Could you check a few things on this model? Use its own coordinates, in mm. A direction names the side the tool comes from. Give positions to 0.01 mm unless a question says otherwise; leave off trailing zeros. Write each loop counter-clockwise with the first axis right and the second up, starting at its lowest first coordinate (ties: lowest second). Pieces come first, ordered by that corner, then holes. Notation, with made-up numbers: M 10,28 L 27,28 A17 cw 27,41 Z; hole C -28.5,-35.75 d2. An arc over 180 degrees is marked long. Use one line per item in the form item = value.
from build123d import *

# Parameters (mm, degrees)
F0_R     = 50.738989
F1_DEPTH = 30
F2_W     = 32.749631
F2_H     = 24.249479
F3_DEPTH = 96.840864
F4_R     = 10


with BuildPart() as f1:
    # F0 (on Front) → F1 (new body)
    with BuildSketch(Plane.XZ):
        Circle(F0_R)
    extrude(amount=F1_DEPTH)

    # F2 (on face) → F3 (cut)
    with BuildSketch(Plane(origin=(0, 0, 0), x_dir=(-1, 0, 0), z_dir=(0, 1, 0))):
        with Locations((16.374816, 12.124739)):
            Rectangle(F2_W, F2_H)
    extrude(amount=-F3_DEPTH, mode=Mode.SUBTRACT)

    # F4
    f4_edges = [f1.edges().sort_by_distance(p)[0] for p in [
        (-50.738989, -30, 0),
    ]]
    fillet(f4_edges, radius=F4_R)


solid = f1.part
1) I want a section at A-A, the plane y = -17. Please give me the cut outline in (x, z), plus the area to 3 significant figures.
Checked values:
outline = C 0,0 d101.48; hole M -32.75,0 L 0,0 L 0,24.25 L -32.75,24.25 Z
area = 7,290 mm2
2) Thinking about a two-plate mould opening in X: for faces 1 (the flat face through (-16, -15, 0)), 2 (the flat face through (8, -30, 1)), 3 (the flat face through (-32.75, -15, 12)), 4 (the cylindrical face through (-10.999, -9.86, -49.532)), which applies, released by +X, released by -X, zero draft, split by the parting line, or undercut?
Checked values:
face_1 = undercut
face_2 = zero draft
face_3 = undercut
face_4 = split by the parting line
3) For faces 5 (the flat face through (-1, 0, -11)), 6 (the flat face through (-16, -15, 24.249)), which set-ups out of +Z, -Z, +X, -X, +Y, -Y let a thin tool reach every point of the face, with its end or its side?
Checked values:
face_5 = +Z, -Z, +X, -X, +Y
face_6 = +Y, -Y
4) If I drill on L1, parallel to Z at x = -23, y = -2.5; L2, parallel to Z at x = -12, y = -17.5; L3, parallel to Z at x = -42.5, y = -24.5, over which ranges is the centre line in solid material (lowest first)?
Checked values:
L1 = -45.23 to 0, 24.25 to 45.23
L2 = -49.3 to 0, 24.25 to 49.3
L3 = -25.71 to 25.71
5) For pin 1 Ø4 at (y, z) = (-18.5, -31.5) entering from -X; pin 2 Ø15 at (x, y) = (-24, -11) entering from +Z; pin 3 Ø5 at (x, y) = (-29.5, -7.5) entering from -Z, each with a flat end and sliding along its axis, tell me the tip position at first contact or that it passes through.
Checked values:
pin_1 = -41.28
pin_2 = 47.98
pin_3 = -42.96
